Geometry: see drawing. Coordinates: mm, zero at the bounding-box minimum. Coordinates: 2 decimals unless noted, no trailing zeros. Write each loop counter-clockwise with the first axis right and the second up, starting at its lowest first coordinate (ties: lowest second). Pieces come first, ordered by that corner, then holes. Notation, with made-up numbers: M 77.5,-29 L 109.5,-29 A32 ccw 109.5,10 Z; hole C 85,66 d8. An arc over 180 degrees is marked long. One line per item, written item: value. Start each with the question number.
Item 1: Cut plane D-D, the plane y = 11.75. Output: boundary loops of the cut face in (x, z) (1 decimal).
Item 2: Ray query, L1, parallel to X at y = 6.5, z = 2.4 (1 decimal); L2, parallel to Y at x = 5.75, z = 1.4; L3, parallel to Y at x = 2.75, z = 1.8 (1 decimal). Return the intervals inside material, ascending. Write a range as from..to.
Item 3: Mould query, pull axis Y, two halves, no side actions, for the marked faces 1, 2, 3 and 4. Classes: released by +Y, released by -Y, zero draft, split by the parting line, or undercut.
Item 4: Cut plane C-C, the plane x = 8.25. Output: boundary loops of the cut face in (y, z) (1 decimal).
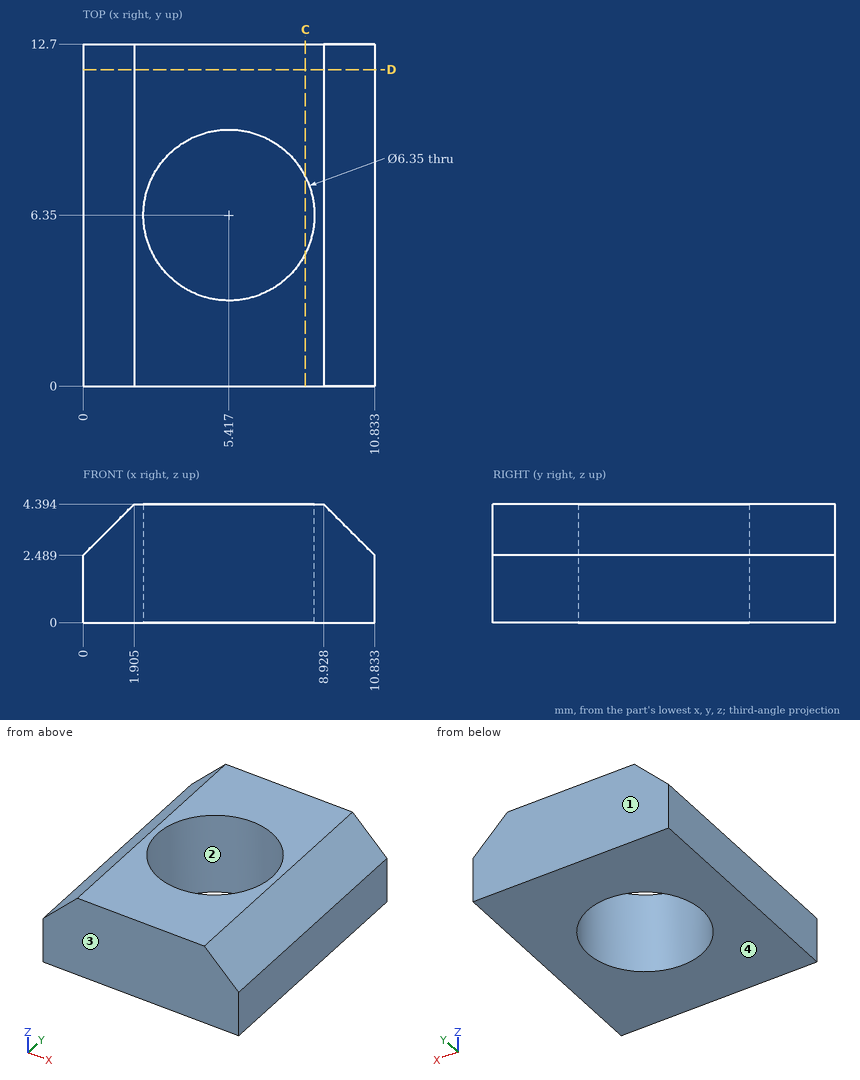
From the geometry:
1. outline: M 0,0 L 10.8,0 L 10.8,2.5 L 8.9,4.4 L 1.9,4.4 L 0,2.5 Z
2. L1: x = 0..2.2, 8.6..10.8
2. L2: y = 0..3.19, 9.51..12.7
2. L3: y = 0..4.6, 8.1..12.7
3. face 1: released by +Y
3. face 2: undercut
3. face 3: released by -Y
3. face 4: zero draft
4. outline: M 0,0 L 4.9,0 L 4.9,4.4 L 0,4.4 Z; M 7.8,0 L 12.7,0 L 12.7,4.4 L 7.8,4.4 Z
